```python
from build123d import *

# Parameters (mm, degrees)
F1_DEPTH        = 33.5
F2_R            = 6
F5_SIZE         = 5
F6_D            = 5.1
F6_CSINK_D      = 10
F6_CSINK_ANGLE  = 90
F7_W            = 8
F7_H            = 25
F8_DEPTH        = 12.5
F9_R            = 12.49999
F12_D           = 4.2
F12_DEPTH       = 13
F12_CSINK_D     = 11.2
F12_CSINK_ANGLE = 90
F12_TIP         = 1.2618073


# Not quite as in the source:
# - a fillet or chamfer is up to 0.001 mm smaller than in the source, because OpenCascade refuses the exact size


with BuildPart() as f1:
    # F0 (on Front) → F1 (new body)
    with BuildSketch(Plane.XZ):
        with BuildLine():
            Line((0, -25.4421804936), (0, -66.931756967))
            Line((0, -66.931756967), (6.3, -66.931756967))
            Line((6.3, -66.931756967), (6.3, -25.4421804936))
            ThreePointArc((6.3, -25.4421804936), (5.7176774776, -14.3308048482), (3.977089958, -3.3411677597))
            Line((3.977089958, -3.3411677597), (-12.8721835275, 75.928431603))
            ThreePointArc((-12.8721835275, 75.928431603), (-20.8378170534, 101.9828448791), (-33.2067360929, 126.2582153279))
            Line((-33.2067360929, 126.2582153279), (-40.38764708, 137.7500751305))
            Line((-40.38764708, 137.7500751305), (-45.7303500858, 134.4115837658))
            Line((-45.7303500858, 134.4115837658), (-38.5494390987, 122.9197239632))
            ThreePointArc((-38.5494390987, 122.9197239632), (-26.6790753372, 99.6228233406), (-19.0345134121, 74.6185879509))
            Line((-19.0345134121, 74.6185879509), (-2.1852399266, -4.6510114118))
            ThreePointArc((-2.1852399266, -4.6510114118), (-0.5478104632, -14.9893341668), (0, -25.4421804936))
        make_face()
    extrude(amount=F1_DEPTH)

    # F2
    f2_edges = [f1.edges().sort_by_distance(p)[0] for p in [
        (-43.058999, -33.5, 136.080829),
        (-43.058999, 0, 136.080829),
    ]]
    fillet(f2_edges, radius=F2_R)

    # F5
    f5_edges = [f1.edges().sort_by_distance(p)[0] for p in [
        (3.15, -33.5, -66.931757),
        (3.15, 0, -66.931757),
    ]]
    chamfer(f5_edges, length=F5_SIZE)

    # F6 (through all)
    with Locations(Plane.YZ.offset(6.3)):
        with Locations((-16.75, -36.631756967), (-16.75, -48.631756967), (-26.75, -60.631756967), (-6.75, -60.631756967)):
            CounterSinkHole(F6_D / 2, F6_CSINK_D / 2, counter_sink_angle=F6_CSINK_ANGLE)

    # F7 (on face) → F8 (join)
    with BuildSketch(Plane(origin=(-3.036646352, 0, -0.6454591076), x_dir=(0, -1, 0), z_dir=(-0.9781476007, 0, -0.2079116908))):
        with Locations((16.75, 19.5)):
            Rectangle(F7_W, F7_H)
    extrude(amount=F8_DEPTH)

    # F9 (radius 12.5 in the source; OpenCascade refuses exactly that, so slightly less here)
    f9_edges = [f1.edges().sort_by_distance(p)[0] for p in [
        (-16.718873, -16.75, 3.602678),
        (-21.916665, -16.75, 28.056368),
    ]]
    fillet(f9_edges, radius=F9_R)

    # F12
    with Locations(Plane(origin=(3.1256835326, 0, 0.6643845446), x_dir=(0, -1, 0), z_dir=(0.9781476007, 0, 0.2079116908))):
        with Locations((16.75, -25.5), (16.75, -13.5)):
            CounterSinkHole(F12_D / 2, F12_CSINK_D / 2, depth=F12_DEPTH, counter_sink_angle=F12_CSINK_ANGLE)
            with Locations((0, 0, -(F12_DEPTH + F12_TIP / 2))):  # 118° drill point
                Cone(0, F12_D / 2, F12_TIP, mode=Mode.SUBTRACT)


solid = f1.part
```
Geometry: final body of the model. Coordinates: model frame, mm. Round coordinates to 2 decimals unless told otherwise and drop trailing zeros. Loops run counter-clockwise (first coordinate to the right, second up) from the corner with the lowest first, then second, coordinate; pieces in that order, holes last. Notation, with made-up numbers: (22, -2) -> (33, -2) arc R24 cw to (33, 11) -> close; hole circle Ø2 at (-32, 16). An arc over 180 degrees is marked (long way). Use one line per item in the form item = value.
Item 1: Cut plane B-B on x = -23.5. Output: boundary loops of the cut face in (y, z), then the cut area to 3 significant figures.
Evaluation:
outline = (-33.5, 91) -> (0, 91) -> (0, 108.18) -> (-33.5, 108.18) -> close
area = 576 mm2
Item 2: Material intervals for probe 1 along Z at (x, y) = (1, -16); probe 2 along X at (y, z) = (-15, -57); probe 3 along X at (y, z) = (-13, 99), sorted ascending.
Evaluation:
probe_1 = -66.93 to -51.07, -46.19 to -39.07, -34.19 to 8.75
probe_2 = 0 to 6.3
probe_3 = -26.43 to -19.67
Item 3: Draft query along Z for faces 1 (the flat face through (3, -17, -66.932)), 2 (the cylindrical face through (1.898, -14.202, -48.52)), 3 (the flat face through (0, -16.5, -45.9)), 4 (the cylindrical face through (-42.19, -31.696, 134.606)). Return one class per face: released by +Z, released by -Z, zero draft, split by the parting line, or undercut.
Evaluation:
face_1 = released by -Z
face_2 = undercut
face_3 = zero draft
face_4 = released by +Z
Item 4: Cut plane A-A on z = 99.5. Output: boundary loops of the cut face in (x, y), then the cut area to 3 significant figures.
Evaluation:
outline = (-26.63, -33.5) -> (-19.86, -33.5) -> (-19.86, 0) -> (-26.63, 0) -> close
area = 227 mm2
Item 5: Contact query for flat-ended pins moving along their axis: pin 1 Ø12 at (x, z) = (-10.5, 24) entering from -Y; pin 2 Ø6 at (y, z) = (-16.75, -36.63) entering from +X; pin 3 Ø5 at (y, z) = (-24.5, -7) entering from +X; pin 4 Ø4 at (x, y) = (-40, -7) entering from -Z. Output: stop coordinate, or through.
Evaluation:
pin_1 = -33.5
pin_2 = 4.3
pin_3 = 5.1
pin_4 = 122.03
